```python
from build123d import *

# Parameters (mm, degrees)
F3_DEPTH = 45.974


with BuildPart() as f1:
    # F0 (on Front) → F1 (revolve)
    with BuildSketch(Plane.XZ):
        with BuildLine():
            Line((0, 6.985), (0, 0))
            Line((0, 0), (36.83, 0))
            Line((36.83, 0), (36.83, 6.985))
            ThreePointArc((36.83, 6.985), (18.415, 8.4328), (0, 6.985))
        make_face()
    revolve(axis=Axis((18.415, 0, 0), (1, 0, 0)))

    # F2 (on face) → F3 (cut)
    with BuildSketch(Plane.YZ.offset(36.83)):
        Polygon((2.54, -2.8575), (2.54, 0), (2.54, 2.8575), (-2.54, 2.8575), (-2.54, 0), (-2.54, -2.8575), align=None)
    extrude(amount=-F3_DEPTH, mode=Mode.SUBTRACT)


solid = f1.part
```
Input: part model. Units: mm. Frame: model coordinates. A direction names the side the tool comes from. Coordinates: 2 decimals unless noted, no trailing zeros. Use one line per item in the form item = value.
Q1. Set-up query: faces 1 (the face through (19, 0, -2.858)), 2 (the face through (36.83, -0.1, -3.01)). Return all of +Z, -Z, +X, -X, +Y, -Y with unobstructed straight access to the full face (end or side cutting, diameter ignored); none if empty.
Answer below:
face_1 = +X, -X
face_2 = +Z, -Z, +X, +Y, -Y
Q2. First-contact query: pin 1 (8 mm diameter, centred on x = 11, z = 4.5, fed in from -Y); pin 2 (5.5 mm diameter, centred on x = 12.5, y = -1, fed in from -Z); pin 3 (1.5 mm diameter, centred on x = 5, y = 6.5, fed in from -Z). Flat tips, straight axial feed; report the tip coordinate or a pass-through.
Answer below:
pin_1 = -8.25
pin_2 = -8.39
pin_3 = -5.08
Q3. Material intervals for probe 1 along Y at (x, z) = (12, -2.75); probe 2 along Z at (x, y) = (3, 1); probe 3 along Z at (x, y) = (13.5, -0.25), sorted ascending. Write a range as from..to.
Answer below:
probe_1 = -7.79..-2.54, 2.54..7.79
probe_2 = -7.35..-2.86, 2.86..7.35
probe_3 = -8.33..-2.86, 2.86..8.33
Q4. Draft query along Z for faces 3 (the face through (19, -2.54, 0)), 4 (the face through (0, -0.1, 3.01)). Return one class per face: released by +Z, released by -Z, zero draft, split by the parting line, or undercut.
Answer below:
face_3 = undercut
face_4 = zero draft
